Here's the drawing with two shaded views (mm, measured from the low corner). I have some questions. A direction names the side the tool comes from. Give positions to 0.01 mm unless a question says otherwise; leave off trailing zeros. Write each loop counter-clockwise with the first axis right and the second up, starting at its lowest first coordinate (ties: lowest second). Pieces come first, ordered by that corner, then holes. Notation, with made-up numbers: (-12, 11.5) - (11, 11.5) arc R14 ccw to (11, 16.5) - close; hole circle Ø3 at (73, 6.25). An arc over 180 degrees is marked (long way). Answer as a JSON object with one key per item and string values. Group by question number.
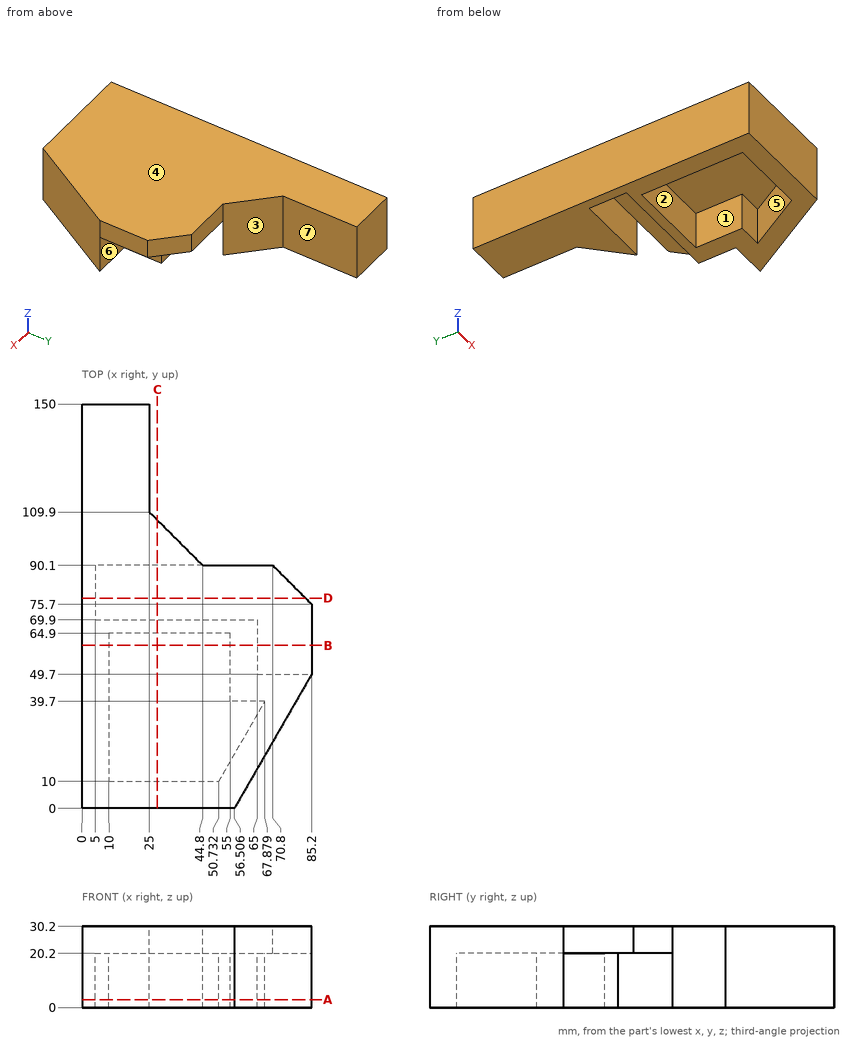
(1) Will these pins go through, and if not, where does the flat tip stop? P1, Ø1.5, axis at x = 33, y = 27, coming from the -Z side; P2, Ø10, axis at y = 61.5, z = 7.5, coming from the +X side; P3, Ø6, axis at x = 73, z = 10.5, coming from the +Y side.
(2) I want a section at C-C, the plane x = 28. Please give me the cut outline in (y, z).
(3) If we mould it in two halves opening along X, with no side actions, what happens to the marked faces 1, 2, 3 and 4? For each: +X half, -X half, draft (parallel to the pull), parting line (faces both ways), or undercut.
(4) I want a section at D-D, the plane y = 78. Please give me the cut outline in (x, z), and give its area (3 significant figures).
(5) I want a section at A-A, the plane z = 3. Please give me the cut outline in (x, y) (1 decimal), and give its area (3 significant figures).
(6) I want a section at B-B, the plane y = 60.5. Please give me the cut outline in (x, z).
(7) I need wall thicknesses on L1, parallel to Y at x = 10.5, z = 9; L2, parallel to Y at x = 50, z = 16; L3, parallel to Y at x = 6, z = 13. Which ranges of each line are inside material? Lowest first, please.
(8) For the marked faces 5, 6 and 7, which set-ups out of +Z, -Z, +X, -X, +Y, -Y let a thin tool reach every point of the face, with its end or its side?
Entries:
{
 "1": {"P1": "z = 20.2", "P2": "x = 65", "P3": "y = 49.7"},
 "2": {"outline": "(0, 0) - (10, 0) - (10, 20.2) - (64.9, 20.2) - (64.9, 0) - (69.9, 0) - (69.9, 20.2) - (90.1, 20.2) - (90.1, 0) - (106.9, 0) - (106.9, 30.2) - (0, 30.2) - close"},
 "3": {"face 1": "undercut", "face 2": "undercut", "face 3": "+X half", "face 4": "draft"},
 "4": {"outline": "(0, 0) - (5, 0) - (5, 20.2) - (82.9, 20.2) - (82.9, 30.2) - (0, 30.2) - close", "area": "930 mm^2"},
 "5": {"outline": "(0, 0) - (56.5, 0) - (85.2, 49.7) - (65, 49.7) - (65, 69.9) - (5, 69.9) - (5, 90.1) - (44.8, 90.1) - (25, 109.9) - (25, 150) - (0, 150) - close; hole (10, 10) - (50.7, 10) - (67.9, 39.7) - (55, 39.7) - (55, 64.9) - (10, 64.9) - close", "area": "4,030 mm^2"},
 "6": {"outline": "(0, 0) - (10, 0) - (10, 20.2) - (55, 20.2) - (55, 0) - (65, 0) - (65, 20.2) - (85.2, 20.2) - (85.2, 30.2) - (0, 30.2) - close"},
 "7": {"L1": "0 to 10, 64.9 to 69.9, 90.1 to 150", "L2": "0 to 10, 64.9 to 69.9", "L3": "0 to 69.9, 90.1 to 150"},
 "8": {"face 5": "-Z", "face 6": "-Z, +X, +Y", "face 7": "+Z, -Z, +X, +Y"}
}
